```python
from build123d import *

# Parameters (mm, degrees)
SKETCH1_W                      = 50.8
SKETCH1_H                      = 19.05
BOSS_EXTRUDE1_DEPTH            = 152.4
CBORE_FOR_M6_SHCS1_D           = 6.6
CBORE_FOR_M6_SHCS1_CBORE_D     = 11
CBORE_FOR_M6_SHCS1_CBORE_DEPTH = 12.35
M6_CLEARANCE_HOLE1_D           = 6.6
M6_CLEARANCE_HOLE2_D           = 6.6


with BuildPart() as part:
    # Sketch1 → Boss-Extrude1 (new body)
    with BuildSketch(Plane.XY):
        with Locations((25.4, 9.525)):
            Rectangle(SKETCH1_W, SKETCH1_H)
    extrude(amount=BOSS_EXTRUDE1_DEPTH)

    # CBORE for M6 SHCS1 (through all)
    with Locations(Plane(origin=(0, 0, 0), x_dir=(-1, 0, 0), z_dir=(0, -1, 0))):
        with Locations((-34.925, -139.7), (-34.925, -107.95), (-15.875, -107.95), (-15.875, -139.7)):
            CounterBoreHole(CBORE_FOR_M6_SHCS1_D / 2, CBORE_FOR_M6_SHCS1_CBORE_D / 2, CBORE_FOR_M6_SHCS1_CBORE_DEPTH)

    # M6 Clearance Hole1 (through all)
    with Locations(Plane.ZY):
        with Locations((9.525, 9.525)):
            Hole(M6_CLEARANCE_HOLE1_D / 2)

    # M6 Clearance Hole2 (through all)
    with Locations(Plane(origin=(0, 0, 0), x_dir=(-1, 0, 0), z_dir=(0, -1, 0))):
        with Locations((-34.925, -25.4), (-15.875, -25.4)):
            Hole(M6_CLEARANCE_HOLE2_D / 2)


solid = part.part
```
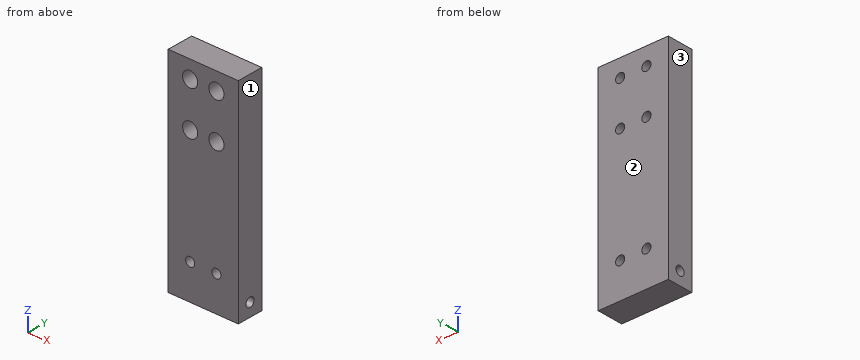
Model file for the job. Use its own axes, mm. Face numbers are marked on the shaded views. Coordinates: 2 decimals unless noted, no trailing zeros. Order: outer loops, then holes, each group sorted by start corner. A loop starts at its lowest first (then second) coordinate and runs counter-clockwise, first axis right, second up. Notation, with made-up numbers: (35.5, -14.5) - (83.5, -14.5) arc R26 ccw to (83.5, 0.5) - close; hole circle Ø7 at (-28.5, -25). An arc over 180 degrees is marked (long way). Return JSON: item names as keys, results as strings. Group by question number.
1) Probe line 1 (X direction, y = 17.5, z = 139.7) (3 decimals); line 2 (X direction, y = 2.5, z = 107.95) (3 decimals); line 3 (Z direction, x = 14.5, y = 12). List the from-to ranges inside material, lowest first. Write a range as from..to.
2) Saw through at D-D, the plane z = 107.95. Write the cut outline in (x, y) (3 decimals).
3) Saw through at C-C, the plane y = 2. Write the cut outline in (x, z) (3 decimals), plus the area to 3 significant figures.
4) Flat gauge pins, fed straight in: P1, Ø4, axis at x = 40, y = 7, coming from the -Z side; P2, Ø10.5, axis at x = 15.875, z = 107.95, coming from the -Y side. Where does each tip first touch, or does it go through?
5) Saw through at A-A, the plane z = 25.4. Write the cut outline in (x, y) (3 decimals).
6) Mould opens along X. For the marked faces 1, 2 and 3 say: released by +X, released by -X, zero draft, split by the parting line, or undercut.
7) Saw through at B-B, the plane x = 14.5. Write the cut outline in (y, z) (3 decimals).
Values found:
{
 "1": {"line 1": "x = 0..12.575, 19.175..31.625, 38.225..50.8", "line 2": "x = 0..10.375, 21.375..29.425, 40.425..50.8", "line 3": "z = 0..7.34, 11.71..22.4, 28.4..102.62, 113.28..134.37, 145.03..152.4"},
 "2": {"outline": "(0, 0) - (10.375, 0) - (10.375, 12.35) - (12.575, 12.35) - (12.575, 19.05) - (0, 19.05) - close; (19.175, 12.35) - (21.375, 12.35) - (21.375, 0) - (29.425, 0) - (29.425, 12.35) - (31.625, 12.35) - (31.625, 19.05) - (19.175, 19.05) - close; (38.225, 12.35) - (40.425, 12.35) - (40.425, 0) - (50.8, 0) - (50.8, 19.05) - (38.225, 19.05) - close"},
 "3": {"outline": "(0, 0) - (50.8, 0) - (50.8, 152.4) - (0, 152.4) - close; hole circle Ø11 at (15.875, 107.95); hole circle Ø11 at (15.875, 139.7); hole circle Ø6.6 at (15.875, 25.4); hole circle Ø11 at (34.925, 107.95); hole circle Ø11 at (34.925, 139.7); hole circle Ø6.6 at (34.925, 25.4)", "area": "7,290 mm²"},
 "4": {"P1": "stops at z = 0", "P2": "stops at y = 12.35"},
 "5": {"outline": "(0, 0) - (12.575, 0) - (12.575, 19.05) - (0, 19.05) - close; (19.175, 0) - (31.625, 0) - (31.625, 19.05) - (19.175, 19.05) - close; (38.225, 0) - (50.8, 0) - (50.8, 19.05) - (38.225, 19.05) - close"},
 "6": {"face 1": "released by +X", "face 2": "zero draft", "face 3": "released by -X"},
 "7": {"outline": "(0, 0) - (19.05, 0) - (19.05, 22.4) - (0, 22.4) - close; (0, 28.4) - (19.05, 28.4) - (19.05, 104.95) - (12.35, 104.95) - (12.35, 102.625) - (0, 102.625) - close; (0, 113.275) - (12.35, 113.275) - (12.35, 110.95) - (19.05, 110.95) - (19.05, 136.7) - (12.35, 136.7) - (12.35, 134.375) - (0, 134.375) - close; (0, 145.025) - (12.35, 145.025) - (12.35, 142.7) - (19.05, 142.7) - (19.05, 152.4) - (0, 152.4) - close; hole circle Ø6.6 at (9.525, 9.525)"}
}
